from build123d import *

# Parameters (mm, degrees)
CUT_EXTRUDE_1_DEPTH      = 4.15
CUT_EXTRUDE_1_DEPTH_BACK = 4.15


with BuildPart() as part:
    # Эскиз1 → Повернуть1 (revolve)
    with BuildSketch(Plane(origin=(0, 0, 0), x_dir=(1, 0, 0), z_dir=(0, 1, 0))):
        Polygon((0, 0), (0, 1.2), (0.3, 1.5), (6.5, 1.5), (6.5, 1.9), (10.8, 1.9), (10.8, 2.3), (11.5, 2.3), (11.5, 3.15), (12.5, 3.15), (12.5, 0), align=None)
    revolve(axis=Axis((-1.842251792, 0, 0), (1, 0, 0)))

    # Эскиз2 → Вырез-Вытянуть1 (cut, two sides)
    with BuildSketch(Plane(origin=(0, 0, 0), x_dir=(1, 0, 0), z_dir=(0, 1, 0))) as cut_extrude_1_sk:
        Polygon((48.434725755, 0.3), (12.5, 0.3), (11.8, 0.3), (11.8, -0.3), (12.5, -0.3), (48.434725755, -0.3), (120.304177266, -0.3), (120.304177266, 0.3), align=None)
    extrude(amount=CUT_EXTRUDE_1_DEPTH, mode=Mode.SUBTRACT)
    extrude(cut_extrude_1_sk.sketch, amount=-CUT_EXTRUDE_1_DEPTH_BACK, mode=Mode.SUBTRACT)


solid = part.part
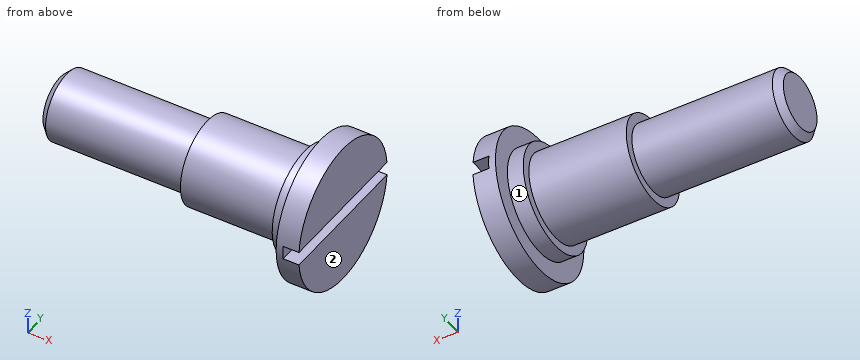
Geometry: final body of the model. Coordinates: model frame, mm. Face numbers are marked on the shaded views. A direction names the side the tool comes from. Round coordinates to 2 decimals unless told otherwise and drop trailing zeros. Loops run counter-clockwise (first coordinate to the right, second up) from the corner with the lowest first, then second, coordinate; pieces in that order, holes last. Notation, with made-up numbers: M -17,82 L 5,82 A18 ccw 5,101 Z; hole C 42,38.25 d7. An arc over 180 degrees is marked long. Put each result on its own line as item: value. Start each with the question number.
(1) Section query A-A (z = 0). Return loops of the section in (x, y), then the cut area to 3 significant figures.
(2) Section query C-C (x = 2.5). Return loops of the section in (y, z).
(3) Section query D-D (x = 9). Return loops of the section in (y, z).
(4) Contact query for flat-ended pins moving along their axis: pin 1 Ø1.5 at (y, z) = (1, 0) entering from -X; pin 2 Ø2 at (x, z) = (9.5, -1.5) entering from +Y; pin 3 Ø2 at (y, z) = (-2, 2) entering from -X. Output: stop coordinate, or through.
(5) Set-up query: the marked faces 1 and 2. Return all of +Z, -Z, +X, -X, +Y, -Y with unobstructed straight access to the full face (end or side cutting, diameter ignored); none if empty.
(6) Material intervals for line 1 along X through (y, z) = (-2.5, -1); line 2 along Y through (x, z) = (5, 0); line 3 along X through (y, z) = (-1.75, 0), sorted ascending. Write a range as [from, to].
(7) Section query B-B (y = 2.75). Return loops of the section in (x, z).
Findings below:
1. outline: M 0,-1.2 L 0.3,-1.5 L 6.5,-1.5 L 6.5,-1.9 L 10.8,-1.9 L 10.8,-2.3 L 11.5,-2.3 L 11.5,-3.15 L 11.8,-3.15 L 11.8,3.15 L 11.5,3.15 L 11.5,2.3 L 10.8,2.3 L 10.8,1.9 L 6.5,1.9 L 6.5,1.5 L 0.3,1.5 L 0,1.2 Z
1. area: 40.9 mm2
2. outline: C 0,0 d3
3. outline: C 0,0 d3.8
4. pin 1: stops at x = 0
4. pin 2: stops at y = 1.83
4. pin 3: stops at x = 6.5
5. face 1: -X
5. face 2: +Z, -Z, +X, +Y, -Y
6. line 1: x = [11.5, 12.5]
6. line 2: y = [-1.5, 1.5]
6. line 3: x = [6.5, 11.8]
7. outline: M 11.5,-1.54 L 12.5,-1.54 L 12.5,-0.3 L 11.8,-0.3 L 11.8,0.3 L 12.5,0.3 L 12.5,1.54 L 11.5,1.54 Z
